```python
from build123d import *

# Parameters (mm, degrees)
BOSS_EXTRUDE1_DEPTH = 1.778
SKETCH2_W           = 8.86
SKETCH2_H           = 13.85
BOSS_EXTRUDE2_DEPTH = 10.9
SKETCH3_R           = 2.3
CUT_EXTRUDE1_DEPTH  = 72.970132694
SKETCH4_W           = 12.192
SKETCH4_H           = 11.684
BOSS_EXTRUDE3_DEPTH = 10.16
SKETCH5_R           = 3.429
BOSS_EXTRUDE4_DEPTH = 3.556
SKETCH6_R           = 3.1496
CUT_EXTRUDE2_DEPTH  = 11.656


with BuildPart() as part:
    # Sketch1 → Boss-Extrude1 (new body)
    with BuildSketch(Plane(origin=(0, 0, 0), x_dir=(1, 0, 0), z_dir=(0, 1, 0))):
        Polygon((-15.075, 69.2), (15.075, 69.2), (15.075, 14.468172401), (16.5, 12), (16.5, 0), (-16.5, 0), (-16.5, 12), (-15.075, 14.468172401), align=None)
    extrude(amount=BOSS_EXTRUDE1_DEPTH)

    # Sketch2 → Boss-Extrude2 (add)
    with BuildSketch(Plane(origin=(0, 1.778, 0), x_dir=(1, 0, 0), z_dir=(0, 1, 0))):
        with Locations((10.17, 6.925)):
            Rectangle(SKETCH2_W, SKETCH2_H)
    extrude(amount=BOSS_EXTRUDE2_DEPTH)

    # Sketch3 → Cut-Extrude1 (cut, through all)
    with BuildSketch(Plane(origin=(0, 1.778, 0), x_dir=(1, 0, 0), z_dir=(0, 1, 0))):
        with Locations(Location((-7.9375, 38.1, 0), (0, 0, 270))):
            Circle(SKETCH3_R)
        with Locations(Location((7.9375, 38.1, 0), (0, 0, 270))):
            Circle(SKETCH3_R)
    extrude(amount=-CUT_EXTRUDE1_DEPTH, mode=Mode.SUBTRACT)

    # Sketch4 → Boss-Extrude3 (add)
    with BuildSketch(Plane(origin=(0, 1.778, 0), x_dir=(1, 0, 0), z_dir=(0, 1, 0))):
        with Locations((-8.88, 5.842)):
            Rectangle(SKETCH4_W, SKETCH4_H)
    extrude(amount=BOSS_EXTRUDE3_DEPTH)

    # Sketch5 → Boss-Extrude4 (add)
    with BuildSketch(Plane.XY):
        with Locations(Location((-8.88, 8.509, 0), (0, 0, 90))):
            Circle(SKETCH5_R)
    extrude(amount=BOSS_EXTRUDE4_DEPTH)

    # Sketch6 → Cut-Extrude2 (cut)
    with BuildSketch(Plane.XY):
        with Locations((10.17, 8.0044)):
            Circle(SKETCH6_R)
    extrude(amount=-CUT_EXTRUDE2_DEPTH, mode=Mode.SUBTRACT)


solid = part.part
```
Geometry check sheet. Reference: the model listing, model coordinates, mm. A direction names the side the tool comes from. Round coordinates to 2 decimals unless told otherwise and drop trailing zeros. Order: outer loops, then holes, each group sorted by start corner. A loop starts at its lowest first (then second) coordinate and runs counter-clockwise, first axis right, second up. Notation, with made-up numbers: (53.25, 21.5) - (86.25, 21.5) arc R15 ccw to (86.25, 28.5) - close; hole circle Ø7 at (58.5, 23.5). An arc over 180 degrees is marked (long way). Use a Markdown table: item, result. Add a question column.
(1) Material ranges on line 1 along X through (y, z) = (1.4, -38.1) (1 decimal); line 2 along Y through (x, z) = (10.17, -2.5); line 3 along Y through (x, z) = (10, -3), recorded low to high. Write a range as [from, to].
(2) Tool access check on faces 4 (the cylindrical face through (-12.28, 8.06, 1.75)), 5 (the flat face through (15.075, 1, -42)), 6 (the flat face through (-9, 11.938, -6)). Record the directions out of +Z, -Z, +X, -X, +Y, -Y that give a thin tool (end or side, any length) a straight path to the whole face; none if there is none.
(3) Sectioned sample at A-A, the plane z = -38.1. Enter the section's corners in (x, y) (1 decimal), and give its area (3 significant figures).
(4) Sectioned sample at C-C, the plane x = 9. Enter the section's corners in (y, z), and give its area (3 significant figures).
(5) Sectioned sample at B-B, the plane y = 3.5. Enter the section's corners in (x, z), and give its area (3 significant figures).
(6) Sectioned sample at D-D, the plane y = 10.5. Enter the section's corners in (x, z), and give its area (3 significant figures).
(7) Release check for a two-part mould opening along Z. For faces 1 (the flat face through (10, 7, -13.85)), 2 (the cylindrical face through (13.174, 8.95, -5.746)), 3 (the cylindrical face through (-7, 1, -36)) record: pulls with the +Z half, pulls with the -Z half, needs draft (parallel to the pull), parting line crosses it, or undercut.
(8) Depth check by flat-ended pin: pin 1 (1.5 mm diameter, centred on y = 3, z = -6, fed in from -X); pin 2 (5 mm diameter, centred on x = 1, y = 7, fed in from -Z); pin 3 (12 mm diameter, centred on x = -7.5, z = -17.5, fed in from +Y); pin 4 (6 mm diameter, centred on y = 4, z = -47, fed in from -X) (3 decimals). Enter the tip coordinate at first touch or a pass-through.
Answers below:
| question | item | result |
|---|---|---|
| 1 | line 1 | [-15.1, -10.2], [-5.6, 5.6], [10.2, 15.1] |
| 1 | line 2 | [0, 4.85], [11.15, 12.68] |
| 1 | line 3 | [0, 4.86], [11.15, 12.68] |
| 2 | face 4 | +Z |
| 2 | face 5 | -Z, +X, +Y, -Y |
| 2 | face 6 | +Z, -Z, -X, +Y |
| 3 | outline | (-15.1, 0) - (-10.2, 0) - (-10.2, 1.8) - (-15.1, 1.8) - close; (-5.6, 0) - (5.6, 0) - (5.6, 1.8) - (-5.6, 1.8) - close; (10.2, 0) - (15.1, 0) - (15.1, 1.8) - (10.2, 1.8) - close |
| 3 | area | 37.2 mm² |
| 4 | outline | (0, -69.2) - (1.78, -69.2) - (1.78, -40.14) - (0, -40.14) - close; (0, -36.06) - (1.78, -36.06) - (1.78, -13.85) - (12.68, -13.85) - (12.68, 0) - (10.93, 0) - (10.93, -11.66) - (5.08, -11.66) - (5.08, 0) - (0, 0) - close |
| 4 | area | 199 mm² |
| 5 | outline | (-14.98, -11.68) - (-2.78, -11.68) - (-2.78, 0) - (-14.98, 0) - close; (5.74, -13.85) - (14.6, -13.85) - (14.6, 0) - (5.74, 0) - close |
| 5 | area | 265 mm² |
| 6 | outline | (-14.98, -11.68) - (-2.78, -11.68) - (-2.78, 0) - (-6.09, 0) - (-6.09, 3.56) - (-11.67, 3.56) - (-11.67, 0) - (-14.98, 0) - close; (5.74, -13.85) - (14.6, -13.85) - (14.6, 0) - (12.09, 0) - (12.09, -11.66) - (8.25, -11.66) - (8.25, 0) - (5.74, 0) - close |
| 6 | area | 240 mm² |
| 7 | face 1 | pulls with the -Z half |
| 7 | face 2 | needs draft |
| 7 | face 3 | undercut |
| 8 | pin 1 | x = -14.98 |
| 8 | pin 2 | through |
| 8 | pin 3 | y = 11.94 |
| 8 | pin 4 | x = -15.075 |
